```python
from build123d import *

# Parameters (mm, degrees)
SKETCH1_R                = 10
BOSS_EXTRUDE1_DEPTH      = 12
SKETCH1_3_R              = 35
SKETCH1_3_R_2            = 20
BOSS_EXTRUDE2_DEPTH      = 50
BOSS_EXTRUDE3_START      = 12
BOSS_EXTRUDE3_DEPTH      = 10
BOSS_EXTRUDE4_DEPTH      = 4
BOSS_EXTRUDE4_DEPTH_BACK = 10
SKETCH5_R                = 15
SKETCH6_R                = 7.5
CUT_EXTRUDE1_DEPTH       = 129.903064355
FILLET1_R                = 8


with BuildPart() as part:
    # Sketch1 → Boss-Extrude1 (new body)
    with BuildSketch(Plane.XY):
        with BuildLine():
            Line((50, 20), (28.722813233, 20))
            ThreePointArc((28.722813233, 20), (33.393850206, 10.480971731), (35, 0))
            ThreePointArc((35, 0), (-10.480971731, -33.393850206), (-28.722813233, 20))
            Line((-28.722813233, 20), (-50, 20))
            ThreePointArc((-50, 20), (-68.47759065, 7.653668647), (-64.142135624, -14.142135624))
            Line((-64.142135624, -14.142135624), (-14.142135624, -64.142135624))
            ThreePointArc((-14.142135624, -64.142135624), (0, -70), (14.142135624, -64.142135624))
            Line((14.142135624, -64.142135624), (64.142135624, -14.142135624))
            ThreePointArc((64.142135624, -14.142135624), (68.47759065, 7.653668647), (50, 20))
        make_face()
        with Locations((0, -50)):
            Circle(SKETCH1_R, mode=Mode.SUBTRACT)
        with Locations((-50, 0)):
            Circle(SKETCH1_R, mode=Mode.SUBTRACT)
        with Locations((50, 0)):
            Circle(SKETCH1_R, mode=Mode.SUBTRACT)
    extrude(amount=BOSS_EXTRUDE1_DEPTH)

    # Sketch1<3> → Boss-Extrude2 (add)
    with BuildSketch(Plane.XY):
        with Locations(Location((0, 0, 0), (0, 0, 145.150095421))):
            Circle(SKETCH1_3_R)
        Circle(SKETCH1_3_R_2, mode=Mode.SUBTRACT)
    extrude(amount=BOSS_EXTRUDE2_DEPTH)

    # Sketch4 → Boss-Extrude3 (add)
    with BuildSketch(Plane(origin=(0, 0, 0), x_dir=(0, 0, -1), z_dir=(1, 0, 0)).offset(BOSS_EXTRUDE3_START)):
        Polygon((-14, 55), (-44, 55), (-44, 35), (-44, 20), (-14, 20), align=None)
    extrude(amount=BOSS_EXTRUDE3_DEPTH)

    # Sketch5 → Boss-Extrude4 (add, two sides: drawn at the far end of the back side and taken through both)
    with BuildSketch(Plane(origin=(22, 0, 0), x_dir=(0, 0, -1), z_dir=(1, 0, 0)).offset(-BOSS_EXTRUDE4_DEPTH_BACK)):
        with Locations((-29, 55)):
            Circle(SKETCH5_R)
    extrude(amount=BOSS_EXTRUDE4_DEPTH + BOSS_EXTRUDE4_DEPTH_BACK)

    # Sketch6 → Cut-Extrude1 (cut, through all)
    with BuildSketch(Plane(origin=(26, 0, 0), x_dir=(0, 0, -1), z_dir=(1, 0, 0))):
        with Locations((-29, 55)):
            Circle(SKETCH6_R)
    extrude(amount=-CUT_EXTRUDE1_DEPTH, mode=Mode.SUBTRACT)

    # Mirror1: part across plane


with BuildPart() as part_1:
    add(part.part)
    add(part.part.mirror(Plane(origin=(0, 0, 0), x_dir=(0, 0, 1), z_dir=(1, 0, 0))))

    # Fillet1
    # the kernel refuses this fillet: 8 mm, written as the material it adds along each edge
    with BuildSketch(Plane(origin=(-28.722813233, 20, 0), x_dir=(-1, 0, 0), z_dir=(0, 0, 1))) as fillet1_piece_1:
        with BuildLine():
            CenterArc((3.911524511, -8), FILLET1_R, 90, 49.370671217)
            ThreePointArc((-2.159980185, -2.790697674), (-1.044795429, -1.422589257), (0, 0))
            Line((0, 0), (3.911524511, 0))
        make_face()
    extrude(amount=12)
    with BuildSketch(Plane(origin=(28.722813233, 20, 0), x_dir=(-0.6120739787659375, 0.7908005086731007, 0), z_dir=(0, 0, 1))) as fillet1_piece_2:
        with BuildLine():
            CenterArc((3.932261699, -7.989827403), FILLET1_R, 92.889712102, 49.370671217)
            Line((-2.394142371, -3.093235573), (0, 0))
            ThreePointArc((0, 0), (1.764476403, -0.04450511), (3.528952806, 0))
        make_face()
    extrude(amount=12)


solid = part_1.part
```
Geometry check sheet. Reference: the model listing, model coordinates, mm. A direction names the side the tool comes from. Coordinates: 2 decimals unless noted, no trailing zeros. Order: outer loops, then holes, each group sorted by start corner. A loop starts at its lowest first (then second) coordinate and runs counter-clockwise, first axis right, second up. Notation, with made-up numbers: (27.25, -24.75) - (33.25, -24.75) arc R15 ccw to (33.25, -8.75) - close; hole circle Ø4 at (-8, 15). An arc over 180 degrees is marked (long way). Answer as a JSON object with one key per item and string values. Group by question number.
Item 1: Scan lines: probe 1 along X at (y, z) = (61, 19); probe 2 along Y at (x, z) = (0, 24); probe 3 along X at (y, z) = (38.5, 34.5). Record each from-to range of solid material in increasing order.
Item 2: Depth check by flat-ended pin: pin 1 Ø11 at (x, y) = (16, 35) entering from +Z; pin 2 Ø11 at (x, y) = (16, 41) entering from -Z; pin 3 Ø8 at (x, z) = (-10.5, 44) entering from +Y; pin 4 Ø12 at (x, z) = (12.5, 9.5) entering from +Y. Enter the tip coordinate at first touch or a pass-through.
Item 3: Draft check along Y on faces 5 (the face through (-4.336, -19.524, 24.65)), 6 (the face through (41, 20, 6)), 7 (the face through (-2.17, -59.76, 5.92)), 8 (the face through (-1, -21, 0)). Enter one of: +Y half, -Y half, draft (parallel to the pull), parting line (faces both ways), or undercut.
Item 4: Sectioned sample at A-A, the plane z = 29. Record the cut outline in (x, y), and give its area (3 significant figures).
Item 5: Sectioned sample at D-D, the plane y = 58. Record the cut outline in (x, z).
Item 6: Sectioned sample at B-B, the plane y = -50. Record the cut outline in (x, z), and give its area (3 significant figures).
Item 7: Tool access check on faces 1 (the face through (-41, 20, 6)), 2 (the face through (17, 44, 14)), 3 (the face through (12, 48, 33)), 4 (the face through (26, 62, 33)). Record the directions out of +Z, -Z, +X, -X, +Y, -Y that give a thin tool (end or side, any length) a straight path to the whole face; none if there is none.
Item 8: Sectioned sample at C-C, the plane x = -57. Record the cut outline in (y, z) (3 decimals), and give its area (3 significant figures).
Resolved:
{
 "1": {"probe 1": "-26 to -12, 12 to 26", "probe 2": "-35 to -20, 20 to 35", "probe 3": "-22 to -12, 12 to 22"},
 "2": {"pin 1": "z = 50", "pin 2": "z = 14", "pin 3": "y = 64.87", "pin 4": "y = 61.54"},
 "3": {"face 5": "undercut", "face 6": "+Y half", "face 7": "undercut", "face 8": "draft"},
 "4": {"outline": "(-26, 40) - (-22, 40) - (-22, 27.22) arc R35 ccw (long way) to (22, 27.22) - (22, 40) - (26, 40) - (26, 47.5) - (12, 47.5) - (12, 32.88) arc R35 ccw to (-12, 32.88) - (-12, 47.5) - (-26, 47.5) - close; (-26, 62.5) - (-12, 62.5) - (-12, 70) - (-26, 70) - close; (12, 62.5) - (26, 62.5) - (26, 70) - (12, 70) - close; hole circle Ø40 at (0, 0)", "area": "3,200 mm^2"},
 "5": {"outline": "(-26, 14.3) - (-12, 14.3) - (-12, 22.13) - (-26, 22.13) - close; (-26, 35.87) - (-12, 35.87) - (-12, 43.7) - (-26, 43.7) - close; (12, 14.3) - (26, 14.3) - (26, 22.13) - (12, 22.13) - close; (12, 35.87) - (26, 35.87) - (26, 43.7) - (12, 43.7) - close"},
 "6": {"outline": "(-28.28, 0) - (-10, 0) - (-10, 12) - (-28.28, 12) - close; (10, 0) - (28.28, 0) - (28.28, 12) - (10, 12) - close", "area": "439 mm^2"},
 "7": {"face 1": "+Z, -Z, -X, +Y", "face 2": "-Z, +X, +Y", "face 3": "+Z, -Z, +Y", "face 4": "+Z, -Z, +X, +Y"},
 "8": {"outline": "(-21.284, 0) - (-7.141, 0) - (-7.141, 12) - (-21.284, 12) - close; (7.141, 0) - (18.735, 0) - (18.735, 12) - (7.141, 12) - close", "area": "309 mm^2"}
}
